Work out the finished part from the listing and answer in its coordinate system (mm). Coordinates: 2 decimals unless noted, no trailing zeros. Loops run counter-clockwise (first coordinate to the right, second up) from the corner with the lowest first, then second, coordinate; pieces in that order, holes last.
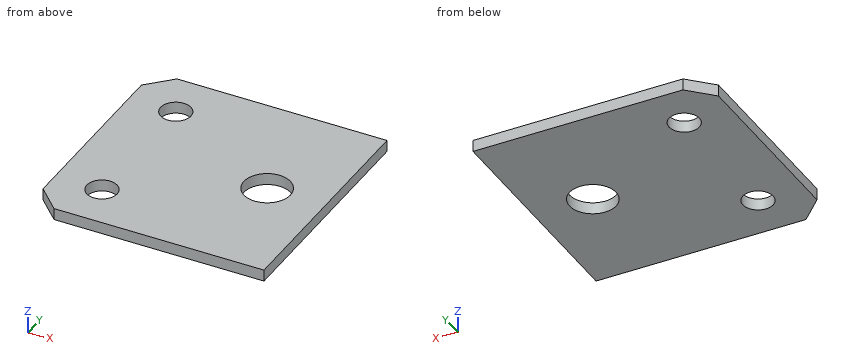
Autodesk Inventor part; units mm, degrees
ref_plane "YZ Plane" through (0, 0, 0) normal (1, 0, 0) x (0, 1, 0)
ref_plane "XZ Plane" through (0, 0, 0) normal (0, 1, 0) x (-1, 0, 0)
ref_plane "XY Plane" through (0, 0, 0) normal (0, 0, 1) x (1, 0, 0)
sketch "Sketch1" plane through (0, 0, 0) normal (0, 0, 1) x (1, 0, 0)
  line L0 (2537.2814, -518.9919) -> (2551.2814, -527.0748)
  line L1 (2551.2814, -527.0748) -> (2565.2814, -518.9919)
  line L2 (2565.2814, -518.9919) -> (2565.2814, -502.826)
  line L3 (2565.2814, -502.826) -> (2551.2814, -494.7431)
  line L4 (2551.2814, -494.7431) -> (2537.2814, -502.826)
  line L5 (2537.2814, -502.826) -> (2537.2814, -518.9919)
  line L6 (2476.2814, -470.9089) -> (2476.2814, -550.9089)
  line L7 (2476.2814, -550.9089) -> (2486.2814, -560.9089)
  line L8 (2486.2814, -560.9089) -> (2576.2814, -560.9089)
  line L9 (2576.2814, -560.9089) -> (2576.2814, -460.9089)
  line L10 (2576.2814, -460.9089) -> (2486.2814, -460.9089)
  line L11 (2486.2814, -460.9089) -> (2476.2814, -470.9089)
  circle A0 centre (2496.2814, -540.9089) radius 6.5
  circle A1 centre (2496.2814, -480.9089) radius 6.5
  circle A2 centre (2551.2814, -510.9089) radius 10
  point P0 (0, 0)
  dimension "d1" = 80
  dimension "d3" = 25
  dimension "d5" = 100
  dimension "d7" = 13
  dimension "d9" = 100
  dimension "d11" = 50
  dimension "d13" = 20
  dimension "d15" = 20
extrude "Extrusion1" add sketch "Sketch1" along normal blind 5 contours L5 L4 L3 L2 L1 L0 | L11 L10 L9 L8 L7 L6
properties part number "ADSK-MH-10042" material "Steel, Mild"
1. A cutting plane is placed at C-C, the plane z = 2.5. Give the vertices of the cut face in (x, y), then the cut area to 3 significant figures.
2. A cutting plane is placed at A-A, the plane x = 2492.5. Give the vertices of the cut face in (y, z).
3. A cutting plane is placed at B-B, the plane x = 2559. Give the vertices of the cut face in (y, z), then the cut area to 3 significant figures.
4. Straight lines are drawn through the part: probe 1 along Y at (x, z) = (2491, 0.2); probe 2 along X at (y, z) = (-546.5, 4.2); probe 3 along X at (y, z) = (-508, 1.45). For each, find the intervals that lie inside material, in ascending order.
5. A cutting plane is placed at D-D, the plane y = -505.5. Give the vertices of the cut face in (x, z).
Answers below:
1. outline: (2476.28, -550.91) - (2486.28, -560.91) - (2576.28, -560.91) - (2576.28, -460.91) - (2486.28, -460.91) - (2476.28, -470.91) - close; hole circle Ø13 at (2496.28, -540.91); hole circle Ø13 at (2496.28, -480.91); hole circle Ø20 at (2551.28, -510.91)
1. area: 9,320 mm2
2. outline: (-560.91, 0) - (-546.2, 0) - (-546.2, 5) - (-560.91, 5) - close; (-535.62, 0) - (-486.2, 0) - (-486.2, 5) - (-535.62, 5) - close; (-475.62, 0) - (-460.91, 0) - (-460.91, 5) - (-475.62, 5) - close
3. outline: (-560.91, 0) - (-517.27, 0) - (-517.27, 5) - (-560.91, 5) - close; (-504.55, 0) - (-460.91, 0) - (-460.91, 5) - (-504.55, 5) - close
3. area: 436 mm2
4. probe 1: y = -560.91 to -544.7, -537.12 to -484.7, -477.12 to -460.91
4. probe 2: x = 2476.28 to 2492.97, 2499.6 to 2576.28
4. probe 3: x = 2476.28 to 2541.71, 2560.85 to 2576.28
5. outline: (2476.28, 0) - (2542.87, 0) - (2542.87, 5) - (2476.28, 5) - close; (2559.69, 0) - (2576.28, 0) - (2576.28, 5) - (2559.69, 5) - close
